Geometry check sheet. Reference: the model listing, model coordinates, mm. Coordinates: 2 decimals unless noted, no trailing zeros. Loops run counter-clockwise (first coordinate to the right, second up) from the corner with the lowest first, then second, coordinate; pieces in that order, holes last. Notation, with made-up numbers: (6.25, 63) - (34.25, 63) arc R5 ccw to (34.25, 70) - close; hole circle Ø4 at (-31, 74.5). An arc over 180 degrees is marked (long way). One line per item, written item: value.
from build123d import *

# Parameters (mm, degrees)
SKETCH1_W           = 23
SKETCH1_H           = 6
SKETCH2_R           = 26
SKETCH2_R_2         = 1
BOSS_EXTRUDE1_DEPTH = 0.5
BOSS_EXTRUDE2_START = 0.5
SKETCH3_R           = 26
BOSS_EXTRUDE2_DEPTH = 0.5
SKETCH4_R           = 1
CUT_EXTRUDE2_DEPTH  = 7


with BuildPart() as part:
    # Sketch1 → Revolve1 (revolve)
    with BuildSketch(Plane(origin=(0, 0, 0), x_dir=(1, 0, 0), z_dir=(0, 1, 0))):
        with BuildLine():
            Line((23, 6), (23, 3))
            ThreePointArc((23, 3), (23.878679656, 5.121320344), (26, 6))
            Line((26, 6), (23, 6))
        make_face()
        with BuildLine():
            Line((23, 3), (23, 0))
            Line((23, 0), (26, 0))
            ThreePointArc((26, 0), (23.878679656, 0.878679656), (23, 3))
        make_face()
        with Locations((11.5, 3)):
            Rectangle(SKETCH1_W, SKETCH1_H)
    revolve(axis=Axis((0, 0, 0), (0, 0, -1)))

    # Sketch2 → Boss-Extrude1 (add)
    with BuildSketch(Plane.XY):
        Circle(SKETCH2_R)
        Circle(SKETCH2_R_2, mode=Mode.SUBTRACT)
    extrude(amount=BOSS_EXTRUDE1_DEPTH)

    # Sketch3 → Boss-Extrude2 (add)
    with BuildSketch(Plane(origin=(0, 0, -6), x_dir=(-1, 0, 0), z_dir=(0, 0, -1)).offset(BOSS_EXTRUDE2_START)):
        with Locations(Location((0, 0, 0), (0, 0, 180))):
            Circle(SKETCH3_R)
    extrude(amount=-BOSS_EXTRUDE2_DEPTH)

    # Sketch4 → Cut-Extrude2 (cut)
    with BuildSketch(Plane(origin=(0, 0, -6.5), x_dir=(-1, 0, 0), z_dir=(0, 0, -1))):
        Circle(SKETCH4_R)
    extrude(amount=-CUT_EXTRUDE2_DEPTH, mode=Mode.SUBTRACT)


solid = part.part
(1) Cross-section at B-B on z = -4. Record the cut outline in (x, y).
Reply:
outline: circle Ø46.34 at (0, 0); hole circle Ø2 at (0, 0)
(2) Cross-section at A-A on z = -1. Record the cut outline in (x, y).
Reply:
outline: circle Ø47.53 at (0, 0); hole circle Ø2 at (0, 0)
(3) Release check for a two-part mould opening along Y. For faces 1 (the face through (0, -1, -3)), 2 (the face through (5, 0, -6.5)), 3 (the face through (-20.633, -15.821, 0.246)) record: pulls with the +Y half, pulls with the -Y half, needs draft (parallel to the pull), parting line crosses it, or undercut.
Reply:
face 1: undercut
face 2: needs draft
face 3: parting line crosses it
(4) Go/stop test with flat-tipped pins: pin 1 Ø1 at (y, z) = (-14, -4) entering from -X; pin 2 Ø3 at (x, z) = (15.5, -3.5) entering from +Y. Record where each tip stops, or that it passes through.
Reply:
pin 1: x = -18.92
pin 2: y = 18.46
(5) Material ranges on probe 1 along X at (y, z) = (0, -2.5); probe 2 along X at (y, z) = (0, -1.25); probe 3 along Y at (x, z) = (0, -3.25), recorded low to high. Write a range as from..to.
Reply:
probe 1: -23.04..-1, 1..23.04
probe 2: -23.56..-1, 1..23.56
probe 3: -23.01..-1, 1..23.01
